Check sheet for the modelled part. Datum: model origin and axes. Units: mm. A direction names the side the tool comes from. Give positions to 0.01 mm unless a question says otherwise; leave off trailing zeros. One line per question, with ' | ' between items. Start each with the question number.
```python
from build123d import *

# Parameters (mm, degrees)
SKETCH1_R           = 23
BOSS_EXTRUDE1_DEPTH = 10
SKETCH2_R           = 18
BOSS_EXTRUDE2_DEPTH = 140
SKETCH3_R           = 21
CUT_EXTRUDE1_DEPTH  = 6
SKETCH4_R           = 17
CUT_EXTRUDE2_DEPTH  = 143
CUT_EXTRUDE3_START  = 10
SKETCH5_R           = 17
CUT_EXTRUDE3_DEPTH  = 10


with BuildPart() as part:
    # Sketch1 → Boss-Extrude1 (new body)
    with BuildSketch(Plane.XY):
        Circle(SKETCH1_R)
    extrude(amount=BOSS_EXTRUDE1_DEPTH)

    # Sketch2 → Boss-Extrude2 (add)
    with BuildSketch(Plane(origin=(0, 0, 0), x_dir=(-1, 0, 0), z_dir=(0, 0, -1))):
        with Locations((-2.9, 4.07)):
            Circle(SKETCH2_R)
    extrude(amount=BOSS_EXTRUDE2_DEPTH)

    # Sketch3 → Cut-Extrude1 (cut)
    with BuildSketch(Plane.XY.offset(10)):
        Circle(SKETCH3_R)
    extrude(amount=-CUT_EXTRUDE1_DEPTH, mode=Mode.SUBTRACT)

    # Sketch4 → Cut-Extrude2 (cut)
    with BuildSketch(Plane.XY.offset(4)):
        with Locations((2.9, 4.07)):
            Circle(SKETCH4_R)
    extrude(amount=-CUT_EXTRUDE2_DEPTH, mode=Mode.SUBTRACT)

    # Sketch5 → Cut-Extrude3 (cut)
    with BuildSketch(Plane.XY.offset(4).offset(CUT_EXTRUDE3_START)):
        with Locations((2.9, 4.07)):
            Circle(SKETCH5_R)
    extrude(amount=-CUT_EXTRUDE3_DEPTH, mode=Mode.SUBTRACT)

    # Sketch6 → Revolve1 (revolve)
    with BuildSketch(Plane(origin=(0, 4.07, 0), x_dir=(1, 0, 0), z_dir=(0, 1, 0))):
        with BuildLine():
            Line((2.9, 142.921547381), (-7.1, 142.921547381))
            ThreePointArc((-7.1, 142.921547381), (-11.369159906, 142.197807517), (-15.1, 140))
            Line((-15.1, 140), (2.9, 140))
            Line((2.9, 140), (2.9, 142.921547381))
        make_face()
    revolve(axis=Axis((2.9, 4.07, -149.3931931), (0, 0, 1)))


solid = part.part
```
Item 1: Scan lines: probe 1 along Y at (x, z) = (2.9, -36); probe 2 along X at (y, z) = (4.5, -53); probe 3 along Z at (x, y) = (13, 7.5). Record each from-to range of solid material in increasing order. Write a range as [from, to].
Item 2: Go/stop test with flat-tipped pins: P1, Ø6, axis at y = -12.5, z = -82, coming from the -X side; P2, Ø6, axis at x = -14.5, z = -94.5, coming from the -Y side; P3, Ø10, axis at x = -15.5, z = -61, coming from the +Y side. Record where each tip stops, or that it passes through.
Item 3: Draft check along Y on faces 1 (the face through (-2.994, 22.804, 4.93)), 2 (the face through (-12.794, -16.652, 7.042)), 3 (the face through (-10, -19, 10)). Enter one of: released by +Y, released by -Y, zero draft, split by the parting line, or undercut.
Item 4: Set-up check for faces 4 (the face through (3, 4, -142.922)), 5 (the face through (6.802, -13.502, -69.02)), 6 (the face through (-0.785, -12.526, -63.457)): record each of +Z, -Z, +X, -X, +Y, -Y from which the full face is reachable in a straight line by a thin tool's end or side.
Reported:
1) probe 1: y = [-13.93, -12.93], [21.07, 22.07] | probe 2: x = [-15.09, -14.09], [19.89, 20.89] | probe 3: z = [-142.91, -139]
2) P1: stops at x = -8.93 | P2: stops at y = -6.73 | P3: stops at y = 16.09
3) face 1: split by the parting line | face 2: undercut | face 3: zero draft
4) face 4: -Z, +X, -X, +Y, -Y | face 5: -Z | face 6: +Z
